The model under review builds one solid part; all positions refer to its coordinate system, in mm. A direction names the side the tool comes from. Coordinates: 2 decimals unless noted, no trailing zeros. Order: outer loops, then holes, each group sorted by start corner. A loop starts at its lowest first (then second) coordinate and runs counter-clockwise, first axis right, second up.
```python
from build123d import *

# Parameters (mm, degrees)
F0_R     = 11.05
F0_R_2   = 7
F1_DEPTH = 0.6
F2_DEPTH = 8.5
F3_R     = 9.3534805389
F4_SIZE  = 0.8
F5_DEPTH = 1.3


with BuildPart() as f1:
    # F0 (on Top) → F1 (new body)
    with BuildSketch(Plane.XY):
        with BuildLine():
            ThreePointArc((-3.5707142143, 12.5), (0, 13), (3.5707142143, 12.5))
            ThreePointArc((3.5707142143, 12.5), (10.3783256064, 17.1711841504), (13, 25))
            ThreePointArc((13, 25), (-7.8288158496, 35.3783256064), (-3.5707142143, 12.5))
        make_face()
        Polygon((4.9074772881, 33.5), (9.8149545762, 25), (4.9074772881, 16.5), (-4.9074772881, 16.5), (-9.8149545762, 25), (-4.9074772881, 33.5), align=None, mode=Mode.SUBTRACT)
        with BuildLine():
            ThreePointArc((13, -25), (10.3783256064, -17.1711841504), (3.5707142143, -12.5))
            ThreePointArc((3.5707142143, -12.5), (0, -13), (-3.5707142143, -12.5))
            ThreePointArc((-3.5707142143, -12.5), (-7.8288158496, -35.3783256064), (13, -25))
        make_face()
        Polygon((-9.8149545762, -25), (-4.9074772881, -16.5), (4.9074772881, -16.5), (9.8149545762, -25), (4.9074772881, -33.5), (-4.9074772881, -33.5), align=None, mode=Mode.SUBTRACT)
        with BuildLine():
            ThreePointArc((3.5707142143, -12.5), (10.3783256064, -7.8288158496), (13, 0))
            ThreePointArc((13, 0), (10.3783256064, 7.8288158496), (3.5707142143, 12.5))
            ThreePointArc((3.5707142143, 12.5), (0, 12), (-3.5707142143, 12.5))
            ThreePointArc((-3.5707142143, 12.5), (-13, 0), (-3.5707142143, -12.5))
            ThreePointArc((-3.5707142143, -12.5), (0, -12), (3.5707142143, -12.5))
        make_face()
        Circle(F0_R, mode=Mode.SUBTRACT)
        Circle(F0_R)
        Circle(F0_R_2, mode=Mode.SUBTRACT)
        Polygon((4.9074772881, 16.5), (9.8149545762, 25), (4.9074772881, 33.5), (-4.9074772881, 33.5), (-9.8149545762, 25), (-4.9074772881, 16.5), align=None)
        Polygon((4.9074772881, -16.5), (-4.9074772881, -16.5), (-9.8149545762, -25), (-4.9074772881, -33.5), (4.9074772881, -33.5), (9.8149545762, -25), align=None)
        with BuildLine():
            ThreePointArc((-3.5707142143, 12.5), (0, 12), (3.5707142143, 12.5))
            ThreePointArc((3.5707142143, 12.5), (0, 13), (-3.5707142143, 12.5))
        make_face()
        with BuildLine():
            ThreePointArc((-3.5707142143, -12.5), (0, -13), (3.5707142143, -12.5))
            ThreePointArc((3.5707142143, -12.5), (0, -12), (-3.5707142143, -12.5))
        make_face()
    extrude(amount=F1_DEPTH)

    # F0 (on Top) → F2 (join)
    with BuildSketch(Plane.XY):
        with BuildLine():
            ThreePointArc((-3.5707142143, 12.5), (0, 13), (3.5707142143, 12.5))
            ThreePointArc((3.5707142143, 12.5), (10.3783256064, 17.1711841504), (13, 25))
            ThreePointArc((13, 25), (-7.8288158496, 35.3783256064), (-3.5707142143, 12.5))
        make_face()
        Polygon((4.9074772881, 33.5), (9.8149545762, 25), (4.9074772881, 16.5), (-4.9074772881, 16.5), (-9.8149545762, 25), (-4.9074772881, 33.5), align=None, mode=Mode.SUBTRACT)
        with BuildLine():
            ThreePointArc((3.5707142143, -12.5), (10.3783256064, -7.8288158496), (13, 0))
            ThreePointArc((13, 0), (10.3783256064, 7.8288158496), (3.5707142143, 12.5))
            ThreePointArc((3.5707142143, 12.5), (0, 12), (-3.5707142143, 12.5))
            ThreePointArc((-3.5707142143, 12.5), (-13, 0), (-3.5707142143, -12.5))
            ThreePointArc((-3.5707142143, -12.5), (0, -12), (3.5707142143, -12.5))
        make_face()
        Circle(F0_R, mode=Mode.SUBTRACT)
        with BuildLine():
            ThreePointArc((-3.5707142143, 12.5), (0, 12), (3.5707142143, 12.5))
            ThreePointArc((3.5707142143, 12.5), (0, 13), (-3.5707142143, 12.5))
        make_face()
        with BuildLine():
            ThreePointArc((-3.5707142143, -12.5), (0, -13), (3.5707142143, -12.5))
            ThreePointArc((3.5707142143, -12.5), (0, -12), (-3.5707142143, -12.5))
        make_face()
        with BuildLine():
            ThreePointArc((13, -25), (10.3783256064, -17.1711841504), (3.5707142143, -12.5))
            ThreePointArc((3.5707142143, -12.5), (0, -13), (-3.5707142143, -12.5))
            ThreePointArc((-3.5707142143, -12.5), (-7.8288158496, -35.3783256064), (13, -25))
        make_face()
        Polygon((-9.8149545762, -25), (-4.9074772881, -16.5), (4.9074772881, -16.5), (9.8149545762, -25), (4.9074772881, -33.5), (-4.9074772881, -33.5), align=None, mode=Mode.SUBTRACT)
    extrude(amount=F2_DEPTH)

    # F3
    f3_edges = [f1.edges().sort_by_distance(p)[0] for p in [
        (3.570714, -12.5, 4.25),
        (3.570714, 12.5, 4.25),
        (-3.570714, 12.5, 4.25),
        (-3.570714, -12.5, 4.25),
    ]]
    fillet(f3_edges, radius=F3_R)

    # F4
    f4_edges = [f1.edges().sort_by_distance(p)[0] for p in [
        (0, -38, 8.5),
        (9.178332, -12.5, 8.5),
        (13, 0, 8.5),
        (9.178332, 12.5, 8.5),
        (0, 38, 8.5),
        (-9.178332, 12.5, 8.5),
        (-13, 0, 8.5),
        (-9.178332, -12.5, 8.5),
        (0, -38, 0),
        (-9.178332, -12.5, 0),
        (-13, 0, 0),
        (-9.178332, 12.5, 0),
        (0, 38, 0),
        (9.178332, 12.5, 0),
        (13, 0, 0),
        (9.178332, -12.5, 0),
    ]]
    chamfer(f4_edges, length=F4_SIZE)

    # F0 (on Top) → F5 (join)
    with BuildSketch(Plane.XY):
        Circle(F0_R)
        Circle(F0_R_2, mode=Mode.SUBTRACT)
    extrude(amount=F5_DEPTH)


solid = f1.part
```
(1) Machinability: for faces 4 (the face through (-12.34, 0.1, 8.36)), 5 (the face through (-7.396, -20.81, 4.495)), which of the approach directions +Z, -Z, +X, -X, +Y, -Y give a long, thin tool a straight path to every point of the face, cutting with its end or side? Answer none if there is none.
A:
face 4: +Z, -X
face 5: +Z
(2) We need section A-A, the plane x = 0. Write out the cut boundary in (y, z), and give its area (3 significant figures).
A:
outline: (-38, 0.8) - (-37.2, 0) - (-7, 0) - (-7, 1.3) - (-11.05, 1.3) - (-11.05, 8.5) - (-16.5, 8.5) - (-16.5, 0.6) - (-33.5, 0.6) - (-33.5, 8.5) - (-37.2, 8.5) - (-38, 7.7) - close; (7, 0) - (37.2, 0) - (38, 0.8) - (38, 7.7) - (37.2, 8.5) - (33.5, 8.5) - (33.5, 0.6) - (16.5, 0.6) - (16.5, 8.5) - (11.05, 8.5) - (11.05, 1.3) - (7, 1.3) - close
area: 199 mm2
(3) Wall thickness on probe 1 along Y at (x, z) = (0.25, 2.75); probe 2 along Y at (x, z) = (-5, 2); probe 3 along Z at (x, y) = (0.75, 31.5): over which ranges is each line inside the solid? List them lowest first.
A:
probe 1: y = -38 to -33.5, -16.5 to -11.05, 11.05 to 16.5, 33.5 to 38
probe 2: y = -37 to -33.34, -16.66 to -9.85, 9.85 to 16.66, 33.34 to 37
probe 3: z = 0 to 0.6
(4) We need section B-B, the plane z = 2.5. Count the separate pieces of the cut face and the enclosed holes in it, and give its area (3 significant figures).
A:
separate pieces: 1
enclosed holes: 3
area: 767 mm2
(5) For pin 1 Ø8 at (x, y) = (-1, -4) entering from +Z; pin 2 Ø1.5 at (x, z) = (-3.5, 2.5) entering from -Y; pin 3 Ø3 at (x, z) = (10, 6.5) entering from -Y, all flat-tipped, find the tip position at first contact; note any pin that passes through.
A:
pin 1: stops at z = 1.3
pin 2: stops at y = -37.71
pin 3: stops at y = -34.84
(6) Draft analysis for pull direction X (two halves, no side actions). For faces 1 (the face through (-2.395, -10.787, 4.85)), 2 (the face through (-13, 0, 4)), 3 (the face through (-8, 1, 0)), state which applies: released by +X, released by -X, zero draft, split by the parting line, or undercut.
A:
face 1: undercut
face 2: released by -X
face 3: zero draft
